from build123d import *

# Parameters (mm, degrees)
BOSS_EXTRUDE1_DEPTH = 1120


with BuildPart() as part:
    # Sketch1 → Boss-Extrude1 (new body)
    with BuildSketch(Plane.XY):
        with BuildLine():
            Line((-45, 80), (45, 80))
            ThreePointArc((45, 80), (52.071067812, 77.071067812), (55, 70))
            Line((55, 70), (55, 65))
            ThreePointArc((55, 65), (52.071067812, 57.928932188), (45, 55))
            Line((45, 55), (20, 55))
            ThreePointArc((20, 55), (12.928932188, 52.071067812), (10, 45))
            Line((10, 45), (10, -55))
            Line((10, -55), (45, -55))
            ThreePointArc((45, -55), (52.071067812, -57.928932188), (55, -65))
            Line((55, -65), (55, -70))
            ThreePointArc((55, -70), (52.071067812, -77.071067812), (45, -80))
            Line((45, -80), (-45, -80))
            ThreePointArc((-45, -80), (-52.071067812, -77.071067812), (-55, -70))
            Line((-55, -70), (-55, -65))
            ThreePointArc((-55, -65), (-52.071067812, -57.928932188), (-45, -55))
            Line((-45, -55), (-20, -55))
            ThreePointArc((-20, -55), (-12.928932188, -52.071067812), (-10, -45))
            Line((-10, -45), (-10, 45))
            ThreePointArc((-10, 45), (-12.928932188, 52.071067812), (-20, 55))
            Line((-20, 55), (-45, 55))
            ThreePointArc((-45, 55), (-52.071067812, 57.928932188), (-55, 65))
            Line((-55, 65), (-55, 70))
            ThreePointArc((-55, 70), (-52.071067812, 77.071067812), (-45, 80))
        make_face()
    extrude(amount=BOSS_EXTRUDE1_DEPTH)


solid = part.part
Geometry check sheet. Reference: the model listing, model coordinates, mm. A direction names the side the tool comes from. Give positions to 0.01 mm unless a question says otherwise; leave off trailing zeros. Order: outer loops, then holes, each group sorted by start corner. A loop starts at its lowest first (then second) coordinate and runs counter-clockwise, first axis right, second up. Notation, with made-up numbers: (49, 23) - (96, 23) arc R27 cw to (96, 41) - close; hole circle Ø1 at (0.5, -37). An arc over 180 degrees is marked (long way). Answer as a JSON object with one key per item and string values.
(1) Cross-section at B-B (z = 728.5). Record the cut outline in (x, y).
Report:
{"outline": "(-55, -70) arc R10 ccw to (-45, -80) - (45, -80) arc R10 ccw to (55, -70) - (55, -65) arc R10 ccw to (45, -55) - (10, -55) - (10, 45) arc R10 cw to (20, 55) - (45, 55) arc R10 ccw to (55, 65) - (55, 70) arc R10 ccw to (45, 80) - (-45, 80) arc R10 ccw to (-55, 70) - (-55, 65) arc R10 ccw to (-45, 55) - (-20, 55) arc R10 cw to (-10, 45) - (-10, -45) arc R10 cw to (-20, -55) - (-45, -55) arc R10 ccw to (-55, -65) - close"}
(2) Draft check along Y on faces 1 (the flat face through (0, -6, 0)), 2 (the flat face through (27, -55, 552)), 3 (the flat face through (-1, 80, 552)), 4 (the flat face through (1, -80, 552)). Enter one of: released by +Y, released by -Y, zero draft, split by the parting line, or undercut.
Report:
{"face 1": "zero draft", "face 2": "undercut", "face 3": "released by +Y", "face 4": "released by -Y"}
(3) Cross-section at C-C (y = -28.5). Record the cut outline in (x, z), then the cut area to 3 significant figures.
Report:
{"outline": "(-10, 0) - (10, 0) - (10, 1120) - (-10, 1120) - close", "area": "22,400 mm^2"}
(4) Cross-section at A-A (x = 31.5). Record the cut outline in (y, z), then the cut area to 3 significant figures.
Report:
{"outline": "(-80, 0) - (-55, 0) - (-55, 1120) - (-80, 1120) - close; (55, 0) - (80, 0) - (80, 1120) - (55, 1120) - close", "area": "56,000 mm^2"}
(5) Depth check by flat-ended pin: pin 1 Ø8 at (y, z) = (6, 729.5) entering from +X; pin 2 Ø3 at (y, z) = (29, 890.5) entering from -X. Enter the tip coordinate at first touch or a pass-through.
Report:
{"pin 1": "x = 10", "pin 2": "x = -10"}
(6) Tool access check on faces 5 (the flat face through (33, 55, 552)), 6 (the flat face through (-33, -55, 552)), 7 (the flat face through (0, -6, 1120)). Record the directions out of +Z, -Z, +X, -X, +Y, -Y that give a thin tool (end or side, any length) a straight path to the whole face; none if there is none.
Report:
{"face 5": "+Z, -Z, +X", "face 6": "+Z, -Z, -X", "face 7": "+Z, +X, -X, +Y, -Y"}
(7) Material ranges on line 1 (Y direction, x = -24.5, z = 496.5); line 2 (X direction, y = 15.5, z = 145.5); line 3 (Y direction, x = -49.5, z = 404), recorded low to high.
Report:
{"line 1": "-80 to -55, 55 to 80", "line 2": "-10 to 10", "line 3": "-78.93 to -56.07, 56.07 to 78.93"}
